```python
from build123d import *

# Parameters (mm, degrees)
SKETCH1_W           = 70
SKETCH1_H           = 12
BOSS_EXTRUDE1_DEPTH = 1.5
SKETCH2_W           = 60
SKETCH2_H           = 6
CUT_EXTRUDE1_DEPTH  = 38.121422387
FILLET1_R           = 10
FILLET2_R           = 5
SKETCH3_W           = 3
SKETCH3_H           = 4
BOSS_EXTRUDE2_DEPTH = 3
SKETCH5_R           = 1.15
CUT_EXTRUDE4_DEPTH  = 10


with BuildPart() as part:
    # Sketch1 → Boss-Extrude1 (new, symmetric)
    with BuildSketch(Plane.XY):
        with Locations((0, 6)):
            Rectangle(SKETCH1_W, SKETCH1_H)
    extrude(amount=BOSS_EXTRUDE1_DEPTH, both=True)

    # Sketch2 → Cut-Extrude1 (cut, through all)
    with BuildSketch(Plane.XY.offset(1.5)):
        with Locations((0, 9)):
            Rectangle(SKETCH2_W, SKETCH2_H)
    extrude(amount=-CUT_EXTRUDE1_DEPTH, mode=Mode.SUBTRACT)

    # Fillet1
    # the kernel refuses this fillet: 10 mm, written as the material it adds along each edge
    with BuildSketch(Plane(origin=(30, 6, 1.5), x_dir=(-1, 0, 0), z_dir=(0, 0, -1))) as fillet1_piece_1:
        with BuildLine():
            CenterArc((9.16515139, 10), FILLET1_R, 203.578178478, 66.421821522)
            Line((0, 6), (-0.183303028, 5.92))
            ThreePointArc((-0.183303028, 5.92), (-0.2, 3), (-0.2, 0))
            Line((-0.2, 0), (0, -0.2))
            Line((0, -0.2), (9.16515139, -0.2))
            Line((9.16515139, -0.2), (9.16515139, 0))
        make_face()
    extrude(amount=3)
    with BuildSketch(Plane(origin=(-30, 6, 1.5), x_dir=(0, 1, 0), z_dir=(0, 0, -1))) as fillet1_piece_2:
        with BuildLine():
            CenterArc((10, 9.16515139), FILLET1_R, 180, 66.421821522)
            Line((0, 9.16515139), (-0.2, 9.16515139))
            Line((-0.2, 9.16515139), (-0.2, 0))
            Line((-0.2, 0), (0, -0.2))
            ThreePointArc((0, -0.2), (3, -0.2), (5.92, -0.183303028))
            Line((5.92, -0.183303028), (6, 0))
        make_face()
    extrude(amount=3)

    # Fillet2
    fillet2_edges = [part.edges().sort_by_distance(p)[0] for p in [
        (-30, 12, 0),
        (30, 12, 0),
    ]]
    fillet(fillet2_edges, radius=FILLET2_R)

    # Sketch3 → Boss-Extrude2 (add)
    with BuildSketch(Plane.XY.offset(1.5)):
        with Locations((36.5, 10)):
            Rectangle(SKETCH3_W, SKETCH3_H)
        with Locations((36.5, 2)):
            Rectangle(SKETCH3_W, SKETCH3_H)
        with Locations((-36.5, 2)):
            Rectangle(SKETCH3_W, SKETCH3_H)
        with Locations((-36.5, 10)):
            Rectangle(SKETCH3_W, SKETCH3_H)
    extrude(amount=-BOSS_EXTRUDE2_DEPTH)

    # Sketch5 → Cut-Extrude4 (cut)
    with BuildSketch(Plane.XY.offset(1.5)):
        with Locations((-0.005546517, 3)):
            Circle(SKETCH5_R)
        with Locations((-6.007488167, 2.994954434)):
            Circle(SKETCH5_R)
        with Locations((5.998183632, 2.997891531)):
            Circle(SKETCH5_R)
        with Locations((17.806168734, 2.989420739)):
            Circle(SKETCH5_R)
        with Locations((23.809898884, 2.98731227)):
            Circle(SKETCH5_R)
        with Locations((-24.075956243, 2.997909584)):
            Circle(SKETCH5_R)
        with Locations((-18.072226094, 2.995801115)):
            Circle(SKETCH5_R)
    extrude(amount=-CUT_EXTRUDE4_DEPTH, mode=Mode.SUBTRACT)


solid = part.part
```
For this review, take the finished solid that the model builds, in its own axes (mm). A direction names the side the tool comes from. Give positions to 0.01 mm unless a question says otherwise; leave off trailing zeros. Order: outer loops, then holes, each group sorted by start corner. A loop starts at its lowest first (then second) coordinate and runs counter-clockwise, first axis right, second up.
1) Take a section at B-B (y = 7.25). Give the boundary of the cut face in (x, z).
2) Take a section at A-A (z = -0.1). Give the boundary of the cut face in (x, y).
3) Insertion check: pin 1 (1.5 mm diameter, centred on y = 5.5, z = -0.5, fed in from -X); pin 2 (1.4 mm diameter, centred on x = -0.01, y = 3, fed in from -Z); pin 3 (1.5 mm diameter, centred on y = 6.5, z = 0.5, fed in from +X); pin 4 (1.5 mm diameter, centred on x = 10.5, z = -0.5, fed in from +Y). Each pin has a flat end and moves straight along its axis. Give the tip position at first contact, or say it passes through.
4) Take a section at C-C (x = 6.5). Give the boundary of the cut face in (y, z).
5) Take a section at D-D (x = 28). Give the boundary of the cut face in (y, z), then the cut area to 3 significant figures.
6) For faces 5 (the face through (-25.249, 7.027, 0.021)), 6 (the face through (-37, 8, 0)), 7 (the face through (36, 4, 0)), list the 3-axis set-ups (+Z, -Z, +X, -X, +Y, -Y) from which the entire face can be reached by the end or side of a thin tool; tool diameter is ignored.
7) Wall thickness on line 1 (Y direction, x = 0, z = 1.25); line 2 (X direction, y = 5.5, z = -1.15): over which ranges is each line inside the solid? List them lowest first.
8) The part is to be moulded in two halves that separate along X. For faces 1 (the face through (38, 10, 0)), 2 (the face through (22.66, 3.04, 0.02)), 3 (the face through (-1, 0, 0)), 4 (the face through (-38, 10, 0)), say which applies: released by +X, released by -X, zero draft, split by the parting line, or undercut.
Derived:
1. outline: (-35, -1.5) - (-25.68, -1.5) - (-25.68, 1.5) - (-35, 1.5) - close; (25.68, -1.5) - (35, -1.5) - (35, 1.5) - (25.68, 1.5) - close
2. outline: (-38, 0) - (38, 0) - (38, 4) - (35, 4) - (35, 8) - (38, 8) - (38, 12) - (32.83, 12) arc R5 ccw to (28.83, 10) arc R10 cw to (20.83, 6) - (-20.83, 6) arc R10 cw to (-28.83, 10) arc R5 ccw to (-32.83, 12) - (-38, 12) - (-38, 8) - (-35, 8) - (-35, 4) - (-38, 4) - close; hole circle Ø2.3 at (-24.08, 3); hole circle Ø2.3 at (-18.07, 3); hole circle Ø2.3 at (-6.01, 2.99); hole circle Ø2.3 at (-0.01, 3); hole circle Ø2.3 at (6, 3); hole circle Ø2.3 at (17.81, 2.99); hole circle Ø2.3 at (23.81, 2.99)
3. pin 1: stops at x = -35
3. pin 2: passes through
3. pin 3: stops at x = 35
3. pin 4: stops at y = 6
4. outline: (0, -1.5) - (1.96, -1.5) - (1.96, 1.5) - (0, 1.5) - close; (4.03, -1.5) - (6, -1.5) - (6, 1.5) - (4.03, 1.5) - close
5. outline: (0, -1.5) - (9.02, -1.5) - (9.02, 1.5) - (0, 1.5) - close
5. area: 27.1 mm2
6. face 5: +Z, -Z, +Y
6. face 6: +Z, -Z, -X
6. face 7: +Z, -Z, +X
7. line 1: y = 0 to 1.85, 4.15 to 6
7. line 2: x = -35 to 35
8. face 1: released by +X
8. face 2: undercut
8. face 3: zero draft
8. face 4: released by -X
